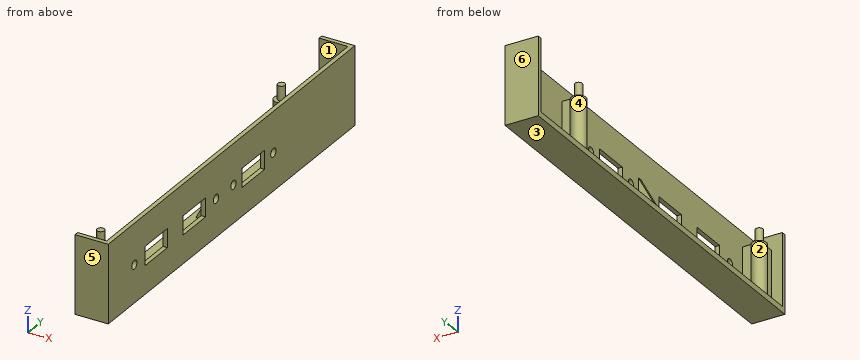
```python
from build123d import *

# Parameters (mm, degrees)
F0_R          = 3.175
F0_R_2        = 1.5875
F1_DEPTH      = 2.54
F2_DEPTH      = 25.4
F3_DEPTH      = 31.75
F5_DEPTH      = 31.75
F5_DEPTH_BACK = 2.54
F7_DEPTH      = 25.4
F8_W          = 16.51
F8_H          = 8.255
F8_R          = 1.905
F9_DEPTH      = 1.905
F12_DEPTH     = 0.9525


with BuildPart() as f1:
    # F0 (on Top) → F1 (new body)
    with BuildSketch(Plane.XY):
        Polygon((6.35, 170.18), (0, 170.18), (-6.35, 170.18), (-6.35, -6.35), (0, -6.35), (6.35, -6.35), align=None)
        Circle(F0_R, mode=Mode.SUBTRACT)
        with Locations((0, 132.08)):
            Circle(F0_R, mode=Mode.SUBTRACT)
        with Locations((0, 132.08)):
            Circle(F0_R)
        with Locations((0, 132.08)):
            Circle(F0_R_2, mode=Mode.SUBTRACT)
        with Locations((0, 132.08)):
            Circle(F0_R_2)
        Circle(F0_R)
        Circle(F0_R_2, mode=Mode.SUBTRACT)
        Circle(F0_R_2)
    extrude(amount=-F1_DEPTH)

    # F0 (on Top) → F2 (join)
    with BuildSketch(Plane.XY):
        with Locations((0, 132.08)):
            Circle(F0_R)
        with Locations((0, 132.08)):
            Circle(F0_R_2, mode=Mode.SUBTRACT)
        with Locations((0, 132.08)):
            Circle(F0_R_2)
        Circle(F0_R_2)
        Circle(F0_R)
        Circle(F0_R_2, mode=Mode.SUBTRACT)
    extrude(amount=F2_DEPTH)

    # F0 (on Top) → F3 (join)
    with BuildSketch(Plane.XY):
        Circle(F0_R_2)
        with Locations((0, 132.08)):
            Circle(F0_R_2)
    extrude(amount=F3_DEPTH)

    # F4 (on Top) → F5 (join, two sides)
    with BuildSketch(Plane.XY) as f5_sk:
        Polygon((-6.35, -6.35), (-6.35, -8.255), (8.255, -8.255), (8.255, 172.085), (-6.35, 172.085), (-6.35, 170.18), (6.35, 170.18), (6.35, -6.35), align=None)
    extrude(amount=F5_DEPTH)
    extrude(f5_sk.sketch, amount=-F5_DEPTH_BACK)

    # F6 (on face) → F7 (join)
    with BuildSketch(Plane.XY):
        with BuildLine():
            Line((6.35, 133.6675), (0, 133.6675))
            ThreePointArc((0, 133.6675), (-1.5875, 132.08), (0, 130.4925))
            Line((0, 130.4925), (6.35, 130.4925))
            Line((6.35, 130.4925), (6.35, 133.6675))
        make_face()
        with BuildLine():
            Line((6.35, 1.5875), (0, 1.5875))
            ThreePointArc((0, 1.5875), (-1.122532, 1.122532), (-1.5875, 0))
            Line((-1.5875, 0), (-1.5875, -6.35))
            Line((-1.5875, -6.35), (1.5875, -6.35))
            Line((1.5875, -6.35), (1.5875, -1.5875))
            Line((1.5875, -1.5875), (6.35, -1.5875))
            Line((6.35, -1.5875), (6.35, 1.5875))
        make_face()
    extrude(amount=F7_DEPTH)

    # F8 (on face) → F9 (cut, through all)
    with BuildSketch(Plane.YZ.offset(8.255)):
        with Locations((26.67, 13.97)):
            Rectangle(F8_W, F8_H)
        with Locations((10.795, 13.97)):
            Circle(F8_R)
        with Locations((54.61, 13.97)):
            Rectangle(F8_W, F8_H)
        with Locations((70.485, 13.97)):
            Circle(F8_R)
        with Locations((97.79, 13.97)):
            Rectangle(F8_W, F8_H)
        with Locations((83.185, 13.97)):
            Circle(F8_R)
        with Locations((112.395, 13.97)):
            Circle(F8_R)
    extrude(amount=-F9_DEPTH, mode=Mode.SUBTRACT)

    # F11 (on offset) → F12 (join, symmetric)
    with BuildSketch(Plane.XZ.offset(-76.835)):
        Polygon((6.35, 19.05), (-3.81, 0), (6.35, 0), align=None)
    extrude(amount=F12_DEPTH, both=True)


solid = f1.part
```
Here's how the part is built. I have some questions about the finished solid (model axes, mm). Face numbers are marked on the shaded views. A direction names the side the tool comes from. Coordinates: 2 decimals unless noted, no trailing zeros. One line per item, written item: value.
1) I'm going to push flat-ended pins straight in: P1, Ø4, axis at x = 2, y = 46, coming from the +Z side; P2, Ø6, axis at y = 95.5, z = 26.5, coming from the -X side; P3, Ø6, axis at x = -3, y = 78, coming from the +Z side. Where does each tip first touch, or does it pass through?
Model answer:
P1: stops at z = 0
P2: stops at x = 6.35
P3: stops at z = 7.13
2) On a 3-axis mill with a long thin cutter (end or side, diameter ignored), from which of +Z, -Z, +X, -X, +Y, -Y can I reach the whole of each face in a straight line? I mean the marked faces 1, 2 and 3. Say none if no direction works.
Model answer:
face 1: +Z, -X
face 2: +Z
face 3: -Z, +X, -X, +Y, -Y
3) I need wall thicknesses on line 1 along Y through (x, z) = (-2.5, 28.5) (3 decimals); line 2 along Y through (x, z) = (0.25, 18) (3 decimals); line 3 along Z through (x, y) = (7, 19). Which ranges of each line are inside material? Lowest first, please.
Model answer:
line 1: y = -8.255 to -6.35, 170.18 to 172.085
line 2: y = -8.255 to 3.165, 128.915 to 135.245, 170.18 to 172.085
line 3: z = -2.54 to 9.84, 18.1 to 31.75
4) We'd pull the mould along Y, two halves only. Please class the marked faces 4, 5 and 6: pulls with the +Y half, pulls with the -Y half, needs draft (parallel to the pull), parting line crosses it, or undercut.
Model answer:
face 4: undercut
face 5: pulls with the -Y half
face 6: pulls with the +Y half
